CAD build for the part. Positions are in the model's coordinates, mm. Round coordinates to 2 decimals unless told otherwise and drop trailing zeros. Order: outer loops, then holes, each group sorted by start corner. A loop starts at its lowest first (then second) coordinate and runs counter-clockwise, first axis right, second up. Notation, with made-up numbers: M 25,-3 L 59,-3 A22 ccw 59,35 Z; hole C 37.25,10.25 d7. An arc over 180 degrees is marked long. Put each result on its own line as item: value.
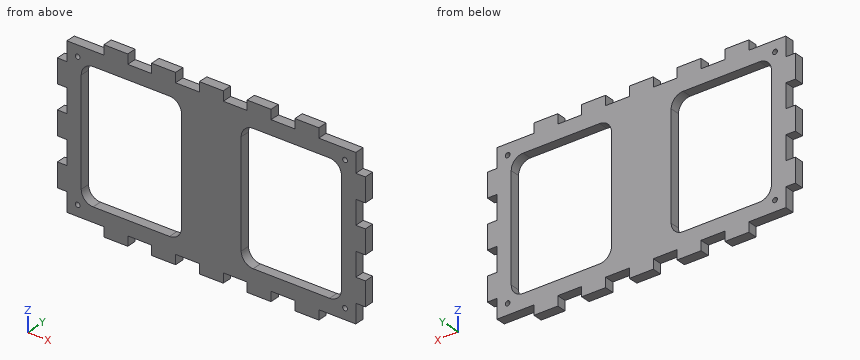
```python
from build123d import *

# Parameters (mm, degrees)
SKETCH1_W           = 121
SKETCH1_H           = 66
BOSS_EXTRUDE1_DEPTH = 4
SKETCH2_W           = 109
SKETCH2_H           = 54
CUT_EXTRUDE1_DEPTH  = 5
FILLET1_R           = 5
SKETCH3_W           = 25
SKETCH3_H           = 54
BOSS_EXTRUDE2_DEPTH = 4
FILLET2_R           = 5
SKETCH4_R           = 1
CUT_EXTRUDE2_DEPTH  = 5
SKETCH5_W           = 10
SKETCH5_H           = 4
BOSS_EXTRUDE3_DEPTH = 4
LPATTERN1_COUNT     = 3
LPATTERN1_PITCH     = 20
LPATTERN1_COL_COUNT = 3
LPATTERN1_COL_PITCH = 20
SKETCH6_W           = 4
SKETCH6_H           = 10
BOSS_EXTRUDE4_DEPTH = 4
LPATTERN2_COUNT     = 2
LPATTERN2_PITCH     = 20
LPATTERN2_COL_COUNT = 2
LPATTERN2_COL_PITCH = 20


with BuildPart() as part:
    # Sketch1 → Boss-Extrude1 (new body)
    with BuildSketch(Plane(origin=(0, 0, 0), x_dir=(1, 0, 0), z_dir=(0, 1, 0))):
        with Locations((60.5, -33)):
            Rectangle(SKETCH1_W, SKETCH1_H)
    extrude(amount=BOSS_EXTRUDE1_DEPTH)

    # Sketch2 → Cut-Extrude1 (cut, through all)
    with BuildSketch(Plane(origin=(0, 4, 0), x_dir=(1, 0, 0), z_dir=(0, 1, 0))):
        with Locations((60.5, -33)):
            Rectangle(SKETCH2_W, SKETCH2_H)
    extrude(amount=-CUT_EXTRUDE1_DEPTH, mode=Mode.SUBTRACT)

    # Fillet1
    fillet1_edges = [part.edges().sort_by_distance(p)[0] for p in [
        (115, 2, 6),
        (115, 2, 60),
        (6, 2, 60),
        (6, 2, 6),
    ]]
    fillet(fillet1_edges, radius=FILLET1_R)

    # Sketch3 → Boss-Extrude2 (add, through all)
    with BuildSketch(Plane(origin=(0, 4, 0), x_dir=(1, 0, 0), z_dir=(0, 1, 0))):
        with Locations((60.5, -33)):
            Rectangle(SKETCH3_W, SKETCH3_H)
    extrude(amount=-BOSS_EXTRUDE2_DEPTH)

    # Fillet2
    fillet2_edges = [part.edges().sort_by_distance(p)[0] for p in [
        (73, 2, 6),
        (73, 2, 60),
        (48, 2, 60),
        (48, 2, 6),
    ]]
    fillet(fillet2_edges, radius=FILLET2_R)

    # Sketch4 → Cut-Extrude2 (cut, through all)
    with BuildSketch(Plane(origin=(0, 4, 0), x_dir=(1, 0, 0), z_dir=(0, 1, 0))):
        with Locations((116.5, -61.5)):
            Circle(SKETCH4_R)
        with Locations((116.5, -4.5)):
            Circle(SKETCH4_R)
        with Locations((4.5, -4.5)):
            Circle(SKETCH4_R)
        with Locations((4.5, -61.5)):
            Circle(SKETCH4_R)
    extrude(amount=-CUT_EXTRUDE2_DEPTH, mode=Mode.SUBTRACT)

    # Sketch5 → Boss-Extrude3 (add, through all)
    with BuildSketch(Plane(origin=(0, 4, 0), x_dir=(1, 0, 0), z_dir=(0, 1, 0))):
        with Locations((60.5, 2)):
            Rectangle(SKETCH5_W, SKETCH5_H)
        with Locations((60.5, -68)):
            Rectangle(SKETCH5_W, SKETCH5_H)
    boss_extrude3 = extrude(amount=-BOSS_EXTRUDE3_DEPTH)

    # LPattern1: Boss-Extrude3 ×3
    with Locations(*[(i * LPATTERN1_PITCH, 0, 0) for i in range(1, LPATTERN1_COUNT)]):
        add(boss_extrude3)

    # LPattern1 col: Boss-Extrude3 ×3
    with Locations(*[(-i * LPATTERN1_COL_PITCH, 0, 0) for i in range(1, LPATTERN1_COL_COUNT)]):
        add(boss_extrude3)

    # Sketch6 → Boss-Extrude4 (add, through all)
    with BuildSketch(Plane(origin=(0, 4, 0), x_dir=(1, 0, 0), z_dir=(0, 1, 0))):
        with Locations((-2, -33)):
            Rectangle(SKETCH6_W, SKETCH6_H)
        with Locations((123, -33)):
            Rectangle(SKETCH6_W, SKETCH6_H)
    boss_extrude4 = extrude(amount=-BOSS_EXTRUDE4_DEPTH)

    # LPattern2: Boss-Extrude4 ×2
    with Locations(*[(0, 0, -i * LPATTERN2_PITCH) for i in range(1, LPATTERN2_COUNT)]):
        add(boss_extrude4)

    # LPattern2 col: Boss-Extrude4 ×2
    with Locations(*[(0, 0, i * LPATTERN2_COL_PITCH) for i in range(1, LPATTERN2_COL_COUNT)]):
        add(boss_extrude4)


solid = part.part
```
Item 1: Band-saw the part on A-A on z = 42. Give the cut face in (x, y).
Answers below:
outline: M 0,0 L 6,0 L 6,4 L 0,4 Z; M 48,0 L 73,0 L 73,4 L 48,4 Z; M 115,0 L 121,0 L 121,4 L 115,4 Z
Item 2: Band-saw the part on D-D on y = 1.9. State how many separate pieces and enclosed holes the cut face has, and give its area (3 significant figures).
Answers below:
separate pieces: 1
enclosed holes: 6
area: 4,120 mm²
Item 3: Probe line 1 along X through (y, z) = (0.3, 29); line 2 along X through (y, z) = (1.85, 44.5); line 3 along Z through (x, y) = (116.5, 1.8). List the from-to ranges inside material, lowest first. Write a range as [from, to].
Answers below:
line 1: [-4, 6], [48, 73], [115, 125]
line 2: [0, 6], [48, 73], [115, 121]
line 3: [0, 3.5], [5.5, 60.5], [62.5, 66]
Item 4: Pin check, flat tips, straight feed: P1, Ø1.2, axis at x = -1.5, y = 1.5, coming from the -Z side; P2, Ø1.2, axis at y = 1.5, z = -2.5, coming from the +X side; P3, Ø1.5, axis at x = 69, z = 39.5, coming from the -Y side; P4, Ø2, axis at y = 1.5, z = 63, coming from the +X side. Stop position of each tip, or through.
Answers below:
P1: z = 8
P2: x = 105.5
P3: y = 0
P4: x = 121
Item 5: Band-saw the part on B-B on x = 22. Give the cut face in (y, z).
Answers below:
outline: M 0,-4 L 4,-4 L 4,6 L 0,6 Z; M 0,60 L 4,60 L 4,70 L 0,70 Z
Item 6: Band-saw the part on C-C on z = 32.5. Give the cut face in (x, y).
Answers below:
outline: M -4,0 L 6,0 L 6,4 L -4,4 Z; M 48,0 L 73,0 L 73,4 L 48,4 Z; M 115,0 L 125,0 L 125,4 L 115,4 Z
